```python
from build123d import *

# Parameters (mm, degrees)
F1_DEPTH = 45
F2_R     = 5
F3_R     = 5
F4_R     = 3
F5_DEPTH = 6
F6_R     = 3
F7_DEPTH = 6


with BuildPart() as f1:
    # F0 (on Front) → F1 (new body)
    with BuildSketch(Plane.XZ):
        with BuildLine():
            Line((17.5, 22.5), (-17.5, 22.5))
            ThreePointArc((-17.5, 22.5), (-21.0355339059, 21.0355339059), (-22.5, 17.5))
            Line((-22.5, 17.5), (-22.5, -17.5))
            ThreePointArc((-22.5, -17.5), (-21.0355339059, -21.0355339059), (-17.5, -22.5))
            Line((-17.5, -22.5), (17.5, -22.5))
            ThreePointArc((17.5, -22.5), (21.0355339059, -21.0355339059), (22.5, -17.5))
            Line((22.5, -17.5), (22.5, 17.5))
            ThreePointArc((22.5, 17.5), (21.0355339059, 21.0355339059), (17.5, 22.5))
        make_face()
    extrude(amount=F1_DEPTH)

    # F2
    f2_edges = [f1.edges().sort_by_distance(p)[0] for p in [
        (0, -45, 22.5),
        (-21.035534, -45, 21.035534),
        (-22.5, -45, 0),
        (-21.035534, -45, -21.035534),
        (0, -45, -22.5),
        (21.035534, -45, -21.035534),
        (22.5, -45, 0),
        (21.035534, -45, 21.035534),
    ]]
    fillet(f2_edges, radius=F2_R)

    # F3
    f3_edges = [f1.edges().sort_by_distance(p)[0] for p in [
        (0, 0, 22.5),
        (-21.035534, 0, 21.035534),
        (-22.5, 0, 0),
        (-21.035534, 0, -21.035534),
        (0, 0, -22.5),
        (21.035534, 0, -21.035534),
        (22.5, 0, 0),
        (21.035534, 0, 21.035534),
    ]]
    fillet(f3_edges, radius=F3_R)

    # F4 (on face) → F5 (cut)
    with BuildSketch(Plane(origin=(-22.5, 0, 0), x_dir=(0, -1, 0), z_dir=(-1, 0, 0))):
        with Locations((22.5, 0)):
            Circle(F4_R)
    extrude(amount=-F5_DEPTH, mode=Mode.SUBTRACT)

    # F6 (on face) → F7 (cut)
    with BuildSketch(Plane.YZ.offset(22.5)):
        with Locations((-31.25, 8.75)):
            Circle(F6_R)
        with Locations((-31.25, 0)):
            Circle(F6_R)
        with Locations((-31.25, -8.75)):
            Circle(F6_R)
        with Locations((-13.75, -8.75)):
            Circle(F6_R)
        with Locations((-13.75, 0)):
            Circle(F6_R)
        with Locations((-13.75, 8.75)):
            Circle(F6_R)
    extrude(amount=-F7_DEPTH, mode=Mode.SUBTRACT)


solid = f1.part
```
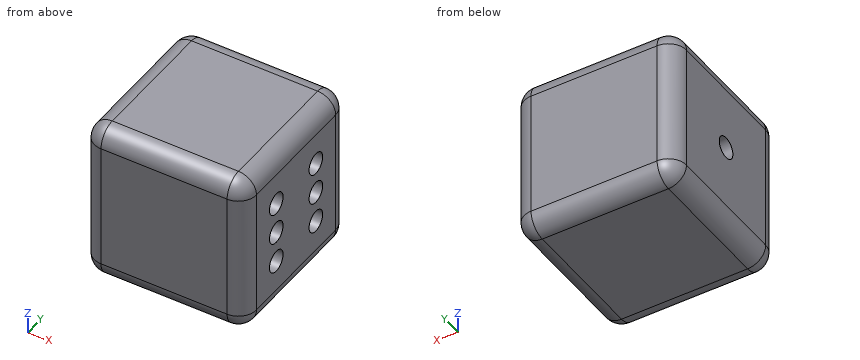
Read the model definition and answer for the solid it produces. Units are mm, in the model's axes. Give positions to 0.01 mm unless a question says otherwise; leave off trailing zeros. Write each loop counter-clockwise with the first axis right and the second up, starting at its lowest first coordinate (ties: lowest second). Pieces come first, ordered by that corner, then holes. Notation, with made-up numbers: (-30, 50) -> (13, 50) arc R25 ccw to (13, 67) -> close; hole circle Ø3 at (11.25, 48). An arc over 180 degrees is marked (long way). Answer in a Markdown table with one row per item.
1) Section B-B on y = -13.75 is taken. Give the vertices of the cut face in (x, z).
Results list:
| item | result |
|---|---|
| outline | (-22.5, -17.5) arc R5 ccw to (-17.5, -22.5) -> (17.5, -22.5) arc R5 ccw to (22.5, -17.5) -> (22.5, -11.75) -> (16.5, -11.75) -> (16.5, -5.75) -> (22.5, -5.75) -> (22.5, -3) -> (16.5, -3) -> (16.5, 3) -> (22.5, 3) -> (22.5, 5.75) -> (16.5, 5.75) -> (16.5, 11.75) -> (22.5, 11.75) -> (22.5, 17.5) arc R5 ccw to (17.5, 22.5) -> (-17.5, 22.5) arc R5 ccw to (-22.5, 17.5) -> close |
2) This flat-tipped pin is pushed along its axis until it touches: pin 1 Ø5.5 at (y, z) = (-31.25, -8.75) entering from +X. Where does it stop, or does it pass through?
Results list:
| item | result |
|---|---|
| pin 1 | x = 16.5 |
3) Section A-A on z = -8.75 is taken. Give the vertices of the cut face in (x, y), plus the area to 3 significant figures.
Results list:
| item | result |
|---|---|
| outline | (-22.5, -40) arc R5 ccw to (-17.5, -45) -> (17.5, -45) arc R5 ccw to (22.5, -40) -> (22.5, -34.25) -> (16.5, -34.25) -> (16.5, -28.25) -> (22.5, -28.25) -> (22.5, -16.75) -> (16.5, -16.75) -> (16.5, -10.75) -> (22.5, -10.75) -> (22.5, -5) arc R5 ccw to (17.5, 0) -> (-17.5, 0) arc R5 ccw to (-22.5, -5) -> close |
| area | 1,930 mm^2 |
4) Straight lines are drawn through the part: line 1 (Z direction, x = 21.35, y = -13.75); line 2 (Z direction, x = 18.95, y = -13.75); line 3 (X direction, y = -12.5, z = 8). For each, find the intervals that lie inside material, in ascending order. Write a range as [from, to].
Results list:
| item | result |
|---|---|
| line 1 | [-20.69, -11.75], [-5.75, -3], [3, 5.75], [11.75, 20.69] |
| line 2 | [-22.29, -11.75], [-5.75, -3], [3, 5.75], [11.75, 22.29] |
| line 3 | [-22.5, 16.5] |
5) Section D-D on z = 10 is taken. Give the vertices of the cut face in (x, y), plus the area to 3 significant figures.
Results list:
| item | result |
|---|---|
| outline | (-22.5, -40) arc R5 ccw to (-17.5, -45) -> (17.5, -45) arc R5 ccw to (22.5, -40) -> (22.5, -33.98) -> (16.5, -33.98) -> (16.5, -28.52) -> (22.5, -28.52) -> (22.5, -16.48) -> (16.5, -16.48) -> (16.5, -11.02) -> (22.5, -11.02) -> (22.5, -5) arc R5 ccw to (17.5, 0) -> (-17.5, 0) arc R5 ccw to (-22.5, -5) -> close |
| area | 1,940 mm^2 |
6) Section C-C on z = 18.5 is taken. Give the vertices of the cut face in (x, y), plus the area to 3 significant figures.
Results list:
| item | result |
|---|---|
| outline | (-22.4, -40) arc R4.9 ccw to (-17.5, -44.9) -> (17.5, -44.9) arc R4.9 ccw to (22.4, -40) -> (22.4, -5) arc R4.9 ccw to (17.5, -0.1) -> (-17.5, -0.1) arc R4.9 ccw to (-22.4, -5) -> close |
| area | 1,990 mm^2 |
